Source: three-view drawing plus pictorial views. Frame: mm from the lowest corner of the part. A direction names the side the tool comes from. Coordinates: 2 decimals unless noted, no trailing zeros. Write each loop counter-clockwise with the first axis right and the second up, starting at its lowest first coordinate (ties: lowest second). Pieces come first, ordered by that corner, then holes. Notation, with made-up numbers: (89, 82) -> (139, 82) arc R9 cw to (139, 96) -> close; hole circle Ø3 at (62, -20.5). An arc over 180 degrees is marked (long way). One line per item, written item: value.
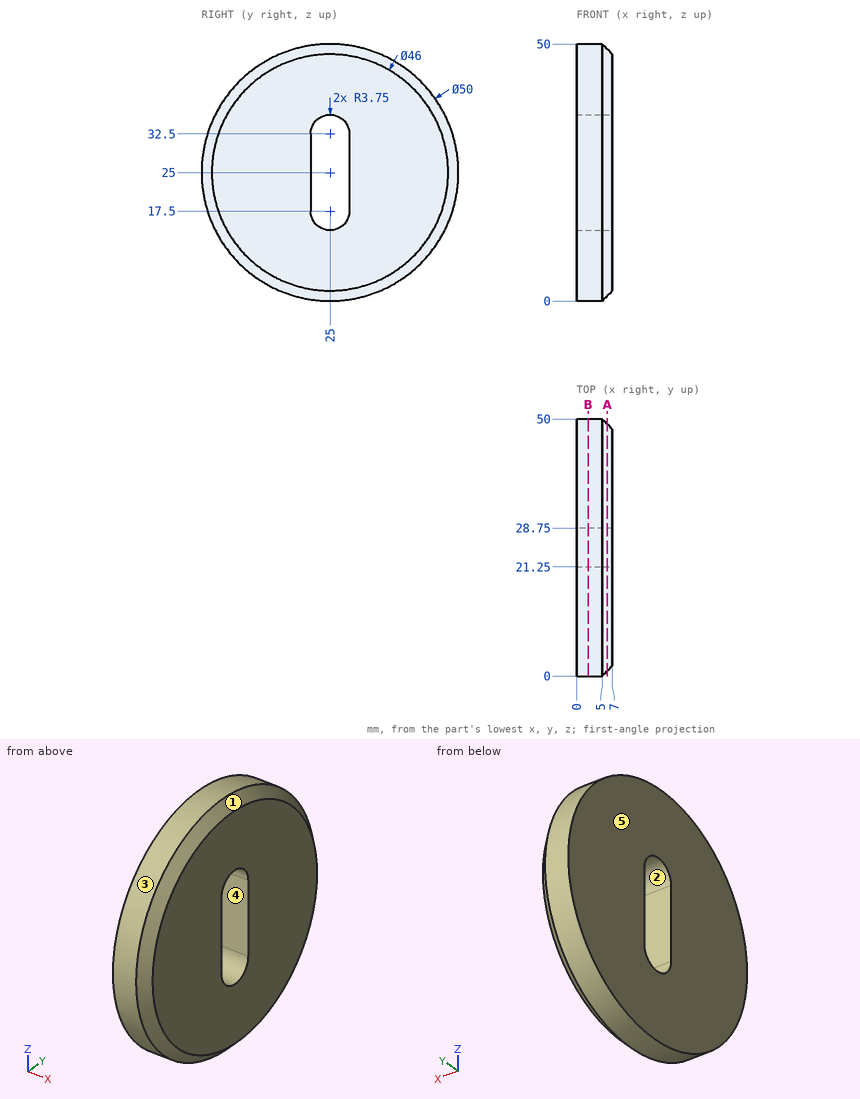
(1) First-contact query: pin 1 (3 mm diameter, centred on x = 1, z = 24.5, fed in from -Y); pin 2 (2 mm diameter, centred on x = 4.5, z = 16.5, fed in from +Y); pin 3 (3 mm diameter, centred on x = 1.5, y = 41.5, fed in from +Z); pin 4 (2 mm diameter, centred on x = 4, y = 22.5, fed in from +Z). Flat tips, straight axial feed; report the tip coordinate or a pass-through.
Responses:
pin 1: stops at y = 0
pin 2: stops at y = 48.85
pin 3: stops at z = 45
pin 4: stops at z = 49.95
(2) Reachability of the marked faces 1 and 2 from +Z, -Z, +X, -X, +Y, -Y: full face, straight path, thin tool, end or side. Return the list, or none.
Responses:
face 1: +X
face 2: +X, -X
(3) Section A-A (x = 6). Return the cut outline in (y, z), then the cut area to 3 significant figures.
Responses:
outline: circle Ø48 at (25, 25); hole (21.25, 17.5) arc R3.75 ccw to (28.75, 17.5) -> (28.75, 32.5) arc R3.75 ccw to (21.25, 32.5) -> close
area: 1,650 mm2
(4) Pull-direction query (Z, two-part tool) for the marked faces 3, 4 and 5; classes: released by +Z, released by -Z, zero draft, split by the parting line, or undercut.
Responses:
face 3: split by the parting line
face 4: undercut
face 5: zero draft
(5) Section B-B (x = 2.25). Return the cut outline in (y, z), then the cut area to 3 significant figures.
Responses:
outline: circle Ø50 at (25, 25); hole (21.25, 17.5) arc R3.75 ccw to (28.75, 17.5) -> (28.75, 32.5) arc R3.75 ccw to (21.25, 32.5) -> close
area: 1,810 mm2
(6) Line query: line 1 (Y direction, x = 0.75, z = 24.5) (3 decimals); line 2 (Z direction, x = 0.75, y = 28); line 3 (Z direction, x = 3, y = 26). Output: solid intervals per line, ascending. Write a range as [from, to].
Responses:
line 1: y = [0.005, 21.25], [28.75, 49.995]
line 2: z = [0.18, 15.25], [34.75, 49.82]
line 3: z = [0.02, 13.89], [36.11, 49.98]
